Input: part model. Units: mm. Frame: model coordinates. A direction names the side the tool comes from. Give positions to 0.01 mm unless a question says otherwise; leave off trailing zeros. Write each loop counter-clockwise with the first axis right and the second up, starting at its lowest first coordinate (ties: lowest second). Pieces come first, ordered by that corner, then holes.
Autodesk Inventor part; units mm, degrees
ref_plane "YZ Plane" through (0, 0, 0) normal (1, 0, 0) x (0, 1, 0)
ref_plane "XZ Plane" through (0, 0, 0) normal (0, 1, 0) x (-1, 0, 0)
ref_plane "XY Plane" through (0, 0, 0) normal (0, 0, 1) x (1, 0, 0)
sketch "Sketch2" plane through (0, 0, 0) normal (0, 0, 1) x (1, 0, 0)
  line L0 (500, -250) -> (160, -250)
  line L1 (-500, -125) -> (-500, 125)
  line L2 (160, 250) -> (500, 250)
  line L3 (500, -250) -> (-500, 250) construction
  line L4 (-500, -250) -> (500, 250) construction
  line L5 (250, 125) -> (250, -125)
  line L6 (500, 250) -> (500, 125)
  line L7 (500, -125) -> (500, -250)
  line L8 (-500, 125) -> (60, 125)
  line L9 (250, 125) -> (500, 125)
  line L10 (-500, -125) -> (60, -125)
  line L11 (250, -125) -> (500, -125)
  line L12 (160, 250) -> (60, 125)
  line L13 (160, -250) -> (60, -125)
  point P0 (0, 0)
  dimension "d0" = 1000
  dimension "d1" = 500
  dimension "d2" = 1000
extrude "Extrusion1" add sketch "Sketch2" along normal blind 125
properties part number "wrench"
Item 1: Section D-D (x = 98). Return loops of the section in (y, z), and give its area (3 significant figures).
Item 2: Section A-A (x = 420.5). Return loops of the section in (y, z).
Item 3: Ray query, line 1 (Y direction, x = 357, z = 34); line 2 (Y direction, x = -371.5, z = 100); line 3 (X direction, y = 132.5, z = 102.5). Return the intervals inside material, ascending.
Item 4: Section B-B (z = 49). Return loops of the section in (x, y), and give its area (3 significant figures).
Item 5: Section C-C (y = -50.5). Return loops of the section in (x, z), and give its area (4 significant figures).
Item 6: Pin query (flat end, axial travel): pin 1 (8 mm diameter, centred on x = 140, z = 50.5, fed in from +Y); pin 2 (1 mm diameter, centred on y = -66.5, z = 95, fed in from +X); pin 3 (5 mm diameter, centred on x = -74, z = 73.5, fed in from -Y). Return the tip coordinate at first contact, or that it passes through.
Item 7: Set-up query: faces 1 (the flat face through (-224, -125, 62)), 2 (the flat face through (-224, 125, 62)), 3 (the flat face through (500, -187, 62)), 4 (the flat face through (373, 125, 62)), 5 (the flat face through (-7, 4, 0)). Return all of +Z, -Z, +X, -X, +Y, -Y with unobstructed straight access to the full face (end or side cutting, diameter ignored); none if empty.
Solved:
1. outline: (-172.5, 0) - (172.5, 0) - (172.5, 125) - (-172.5, 125) - close
1. area: 43,100 mm2
2. outline: (-250, 0) - (-125, 0) - (-125, 125) - (-250, 125) - close; (125, 0) - (250, 0) - (250, 125) - (125, 125) - close
3. line 1: y = -250 to -125, 125 to 250
3. line 2: y = -125 to 125
3. line 3: x = 66 to 500
4. outline: (-500, -125) - (60, -125) - (160, -250) - (500, -250) - (500, -125) - (250, -125) - (250, 125) - (500, 125) - (500, 250) - (160, 250) - (60, 125) - (-500, 125) - close
4. area: 285,000 mm2
5. outline: (-500, 0) - (250, 0) - (250, 125) - (-500, 125) - close
5. area: 93,750 mm2
6. pin 1: stops at y = 230
6. pin 2: stops at x = 250
6. pin 3: stops at y = -125
7. face 1: +Z, -Z, -X, -Y
7. face 2: +Z, -Z, -X, +Y
7. face 3: +Z, -Z, +X, +Y, -Y
7. face 4: +Z, -Z, +X
7. face 5: -Z, +X, -X, +Y, -Y
